from build123d import *

# Parameters (mm, degrees)
SKETCH2_W      = 0.6
SKETCH2_H      = 1.518456807
EXTRUDE1_DEPTH = 1.27
SKETCH3_W      = 1.103174595
SKETCH3_H      = 0.588939024
EXTRUDE2_DEPTH = 1.27
CHAMFER1_SIZE  = 0.254


with BuildPart() as part:
    # Sketch1 → Revolve1 (revolve)
    with BuildSketch(Plane(origin=(0, 0, 0), x_dir=(1, 0, 0), z_dir=(0, 1, 0))):
        with BuildLine():
            Line((0, 0), (0, 7.5))
            ThreePointArc((0, 7.5), (1.059481005, 7.319945729), (2, 6.8))
            Line((2, 6.8), (2, 6))
            Line((2, 6), (1, 6))
            Line((1, 6), (1, 0))
            Line((1, 0), (0, 0))
        make_face()
    revolve(axis=Axis((0, 0, 0), (0, 0, -1)))

    # Sketch2 → Extrude1 (cut, symmetric)
    with BuildSketch(Plane(origin=(0, 0, 0), x_dir=(1, 0, 0), z_dir=(0, 1, 0))):
        with Locations((0, 7.559228404)):
            Rectangle(SKETCH2_W, SKETCH2_H)
    extrude(amount=EXTRUDE1_DEPTH, both=True, mode=Mode.SUBTRACT)

    # Sketch3 → Extrude2 (cut, symmetric)
    with BuildSketch(Plane(origin=(0, 0, 0), x_dir=(0, 0, -1), z_dir=(1, 0, 0))):
        with Locations((7.351587298, 0)):
            Rectangle(SKETCH3_W, SKETCH3_H)
    extrude(amount=EXTRUDE2_DEPTH, both=True, mode=Mode.SUBTRACT)

    # Chamfer1
    chamfer1_edges = [part.edges().sort_by_distance(p)[0] for p in [
        (-1, 0, 0),
    ]]
    chamfer(chamfer1_edges, length=CHAMFER1_SIZE)


solid = part.part
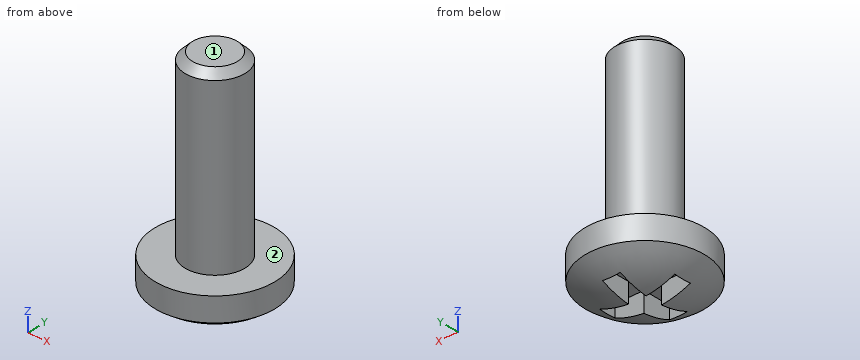
Read the model definition and answer for the solid it produces. Units are mm, in the model's axes. Face numbers are marked on the shaded views. A direction names the side the tool comes from. Give positions to 0.01 mm unless a question says otherwise; leave off trailing zeros. Write each loop counter-clockwise with the first axis right and the second up, starting at its lowest first coordinate (ties: lowest second). Pieces come first, ordered by that corner, then holes. Notation, with made-up numbers: M 62,-22 L 91,-22 A19 cw 91,-9 Z; hole C 12.25,70 d1. An arc over 180 degrees is marked long. One line per item, written item: value. Start each with the question number.
(1) Find section A-A (x = 0). Determine the outline of the cut face in (y, z), plus the area to 3 significant figures.
(2) Find the intervals of material crossed by line 1 (X direction, y = 0, z = -1.5); line 2 (Z direction, x = -0.55, y = 0.2); line 3 (Z direction, x = 0.95, y = 1.05), in increasing order.
(3) Find section D-D (y = 1.1). Determine the outline of the cut face in (x, z), plus the area to 3 significant figures.
(4) Flat-ended cylindrical pins translate along their axes: pin 1 Ø2 at (x, y) = (-0.5, 0) entering from +Z; pin 2 Ø0.5 at (x, z) = (0.5, -7) entering from -Y; pin 3 Ø2 at (y, z) = (1, -5.5) entering from -X; pin 4 Ø2 at (y, z) = (-1, -2.5) entering from -X. Find the tip coordinate at first contact, or state that the pin passes through.
(5) Find section C-C (z = -6.5). Determine the outline of the cut face in (x, y), plus the area to 3 significant figures.
(6) A tool of negligible diameter and unlimited length cuts with its end or side. For the marked faces 1 and 2, from which of +Z, -Z, +X, -X, +Y, -Y can it reach the whole face along a straight path? Write none if from no direction.
Results below:
1. outline: M -2,-6.8 A3.21 ccw -1.27,-7.24 L -1.27,-6.8 L 1.27,-6.8 L 1.27,-7.24 A3.21 ccw 2,-6.8 L 2,-6 L 1,-6 L 1,-0.25 L 0.75,0 L -0.75,0 L -1,-0.25 L -1,-6 L -2,-6 Z
1. area: 15.5 mm^2
2. line 1: x = -1 to 1
2. line 2: z = -6.8 to 0
2. line 3: z = -7.17 to -6
3. outline: M -1.67,-6.8 A3.01 ccw -0.3,-7.29 L -0.3,-6.8 L 0.3,-6.8 L 0.3,-7.29 A3.01 ccw 1.67,-6.8 L 1.67,-6 L -1.67,-6 Z
3. area: 3.52 mm^2
4. pin 1: stops at z = 0
4. pin 2: stops at y = -1.97
4. pin 3: stops at x = -2
4. pin 4: stops at x = -1
5. outline: C 0,0 d4
5. area: 12.6 mm^2
6. face 1: +Z, +X, -X, +Y, -Y
6. face 2: +Z
